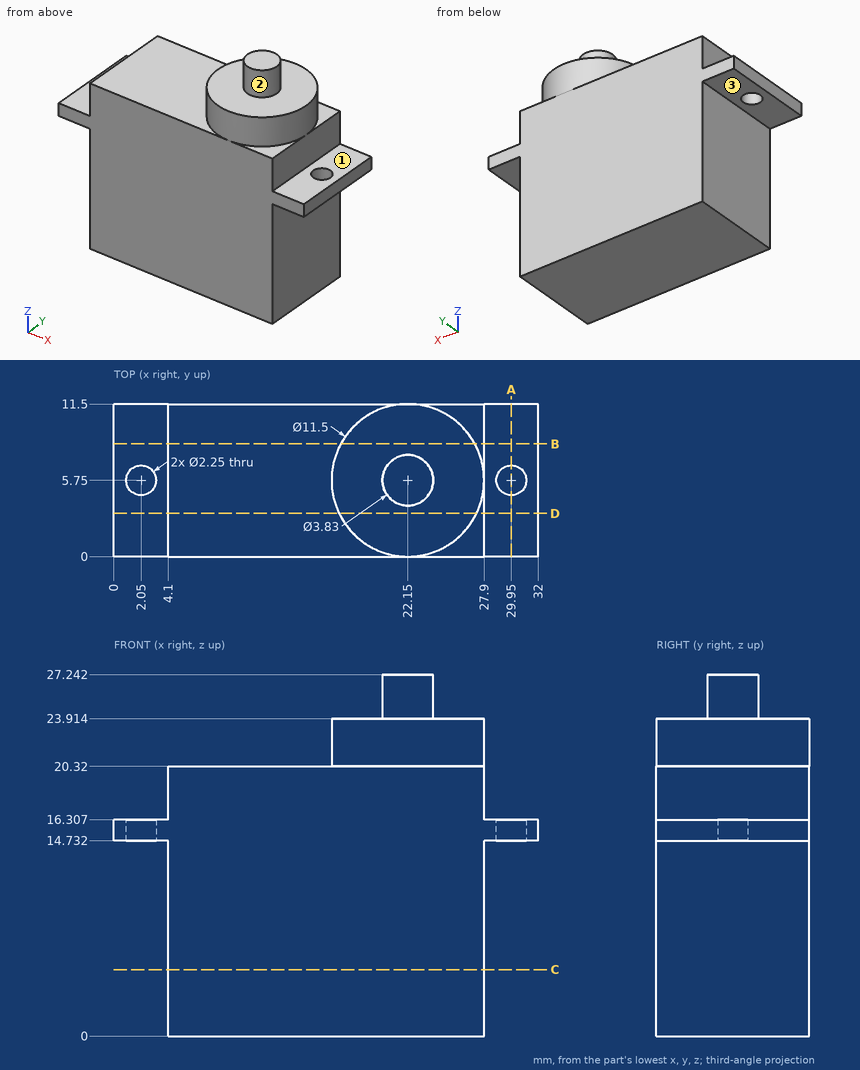
For this review, use the dimensioned drawing (mm, ordinates from the lowest corner) and the shaded views. A direction names the side the tool comes from. Coordinates: 2 decimals unless noted, no trailing zeros. Write each loop counter-clockwise with the first axis right and the second up, starting at its lowest first coordinate (ties: lowest second). Pieces come first, ordered by that corner, then holes. Notation, with made-up numbers: (71, 51) - (84, 51) arc R24 cw to (84, 86) - close; hole circle Ø5 at (-3.75, 63). An arc over 180 degrees is marked (long way). Answer as a JSON object with one key per item and string values. Group by question number.
1. Add section B-B (y = 8.5). Give the boundary of the cut face in (x, z) (1 decimal).
2. Add section D-D (y = 3.25). Give the boundary of the cut face in (x, z) (1 decimal), plus the area to 3 significant figures.
3. Add section C-C (z = 5). Give the boundary of the cut face in (x, y).
4. Clearance check with flat-ended pins moving along their axes: pin 1 Ø1.7 at (x, y) = (24.5, 3.5) entering from +Z; pin 2 Ø1.2 at (y, z) = (8.5, 18.5) entering from +X; pin 3 Ø2 at (x, y) = (2, 3.5) entering from -Z. State where each tip first meets the part, or that it passes through.
5. Machinability: for the marked faces 1, 2 and 3, which of the approach directions +Z, -Z, +X, -X, +Y, -Y give a long, thin tool a straight path to every point of the face, cutting with its end or side? Answer none if there is none.
6. Add section A-A (x = 29.95). Give the boundary of the cut face in (y, z) (1 decimal).
7. To check wall thickness, follow probe 1 along Y at (x, z) = (2.05, 15.9) (1 decimal); probe 2 along X at (y, z) = (6.25, 7); probe 3 along Z at (x, y) = (4, 8). State the ranges of each line that lie inside material, in increasing order.
Findings:
{
 "1": {"outline": "(0, 14.7) - (4.1, 14.7) - (4.1, 0) - (27.9, 0) - (27.9, 14.7) - (32, 14.7) - (32, 16.3) - (27.9, 16.3) - (27.9, 20.3) - (27.2, 20.3) - (27.2, 23.9) - (17.1, 23.9) - (17.1, 20.3) - (4.1, 20.3) - (4.1, 16.3) - (0, 16.3) - close"},
 "2": {"outline": "(0, 14.7) - (4.1, 14.7) - (4.1, 0) - (27.9, 0) - (27.9, 14.7) - (32, 14.7) - (32, 16.3) - (27.9, 16.3) - (27.9, 20.3) - (27.3, 20.3) - (27.3, 23.9) - (17, 23.9) - (17, 20.3) - (4.1, 20.3) - (4.1, 16.3) - (0, 16.3) - close", "area": "534 mm²"},
 "3": {"outline": "(4.1, 0) - (27.9, 0) - (27.9, 11.5) - (4.1, 11.5) - close"},
 "4": {"pin 1": "z = 23.91", "pin 2": "x = 27.9", "pin 3": "z = 14.73"},
 "5": {"face 1": "+Z, +X, +Y, -Y", "face 2": "+Z", "face 3": "-Z, -X, +Y, -Y"},
 "6": {"outline": "(0, 14.7) - (4.6, 14.7) - (4.6, 16.3) - (0, 16.3) - close; (6.9, 14.7) - (11.5, 14.7) - (11.5, 16.3) - (6.9, 16.3) - close"},
 "7": {"probe 1": "0 to 4.6, 6.9 to 11.5", "probe 2": "4.1 to 27.9", "probe 3": "14.73 to 16.31"}
}
